Work out the finished part from the listing and answer in its coordinate system (mm). Face numbers are marked on the shaded views. A direction names the side the tool comes from. Round coordinates to 2 decimals unless told otherwise and drop trailing zeros. Order: outer loops, then holes, each group sorted by start corner. A loop starts at its lowest first (then second) coordinate and runs counter-clockwise, first axis right, second up. Notation, with made-up numbers: M 13,67.25 L 62,67.25 A30 ccw 62,97.25 Z; hole C 8,18.5 d8. An arc over 180 degrees is marked long. Answer as a JSON object with one key per item and string values. Group by question number.
from build123d import *

# Parameters (mm, degrees)
F0_R        = 1.7
F0_R_2      = 1.6
F1_DEPTH    = 10.4
F2_W        = 12.7
F2_H        = 2.7
F2_W_2      = 4
F2_H_2      = 1.35
F3_DEPTH    = 28
F4_W        = 12
F4_H        = 1.35
F5_DEPTH    = 6.2
F6_T1_DEPTH = 23.9048285752
F7_R        = 0.762


# Not quite as in the source:
# - a fillet or chamfer that OpenCascade refuses, or shapes differently, is made with other operations: its cross-section is extruded or revolved along the edge and cut away or added
# - a feature names something its author has since deleted; it is built from what else it names


with BuildPart() as f1:
    # F0 (on Top) → F1 (new body)
    with BuildSketch(Plane.XY):
        with BuildLine():
            Line((3.3782, 0), (0, 0))
            Line((0, 0), (0, -15.8))
            Line((0, -15.8), (15, -15.8))
            Line((15, -15.8), (15, -19.8))
            Line((15, -19.8), (27, -19.8))
            Line((27, -19.8), (27, -19))
            Line((27, -19), (15.8, -19))
            Line((15.8, -19), (15.8, -15.8))
            Line((15.8, -15.8), (28, -15.8))
            Line((28, -15.8), (28, -11))
            Line((28, -11), (40, -11))
            Line((40, -11), (40, -10.2))
            Line((40, -10.2), (28, -10.2))
            Line((28, -10.2), (28, -5.6))
            Line((28, -5.6), (40, -5.6))
            Line((40, -5.6), (40, -4.8))
            Line((40, -4.8), (28, -4.8))
            Line((28, -4.8), (28, 0))
            Line((28, 0), (6.1722, 0))
            Line((6.1722, 0), (6.1722, 1.345))
            ThreePointArc((6.1722, 1.345), (4.7752, 2.742), (3.3782, 1.345))
            Line((3.3782, 1.345), (3.3782, 0))
        make_face()
        with Locations((3.1, -13)):
            Circle(F0_R, mode=Mode.SUBTRACT)
        with Locations((25.3, -2.7)):
            Circle(F0_R_2, mode=Mode.SUBTRACT)
    extrude(amount=F1_DEPTH)

    # F2 (on face) → F3 (cut, through all)
    with BuildSketch(Plane(origin=(0, 0, 0), x_dir=(0, -1, 0), z_dir=(-1, 0, 0))):
        with Locations((-6.35, 9.05)):
            Rectangle(F2_W, F2_H)
        with Locations((-6.35, 1.35)):
            Rectangle(F2_W, F2_H)
        with Locations((17.8, 9.725)):
            Rectangle(F2_W_2, F2_H_2)
        with Locations((17.8, 0.675)):
            Rectangle(F2_W_2, F2_H_2)
    extrude(amount=-F3_DEPTH, mode=Mode.SUBTRACT)

    # F4 (on face) → F5 (cut, through all)
    with BuildSketch(Plane(origin=(0, -4.8, 0), x_dir=(-1, 0, 0), z_dir=(0, 1, 0))):
        with Locations((-34, 9.725)):
            Rectangle(F4_W, F4_H)
        with Locations((-34, 0.675)):
            Rectangle(F4_W, F4_H)
    extrude(amount=-F5_DEPTH, mode=Mode.SUBTRACT)

    # F6: fillet of radius 2.7 on 2 edges, made by hand

    # F6_s2 → F6_t1 (cut)
    with BuildSketch(Plane.XY.offset(-6.7524142876)):
        with BuildLine():
            ThreePointArc((25.2990343146, -15.8004), (27.2091883092, -15.0091883092), (28.0004, -13.0990343146))
            Line((28.0004, -13.0990343146), (28.2705365685, -13.0990343146))
            ThreePointArc((28.2705365685, -13.0990343146), (28.2701365685, -14.4495171573), (28.2701365685, -15.8))
            Line((28.2701365685, -15.8), (28, -16.0701365685))
            ThreePointArc((28, -16.0701365685), (26.6495171573, -16.0701365685), (25.2990343146, -16.0705365685))
            Line((25.2990343146, -16.0705365685), (25.2990343146, -15.8004))
        make_face()
    extrude(amount=F6_T1_DEPTH, mode=Mode.SUBTRACT)

    # F7
    f7_edges = [f1.edges().sort_by_distance(p)[0] for p in [
        (28, 0, 5.2),
        (0, -15.8, 5.2),
    ]]
    fillet(f7_edges, radius=F7_R)


solid = f1.part
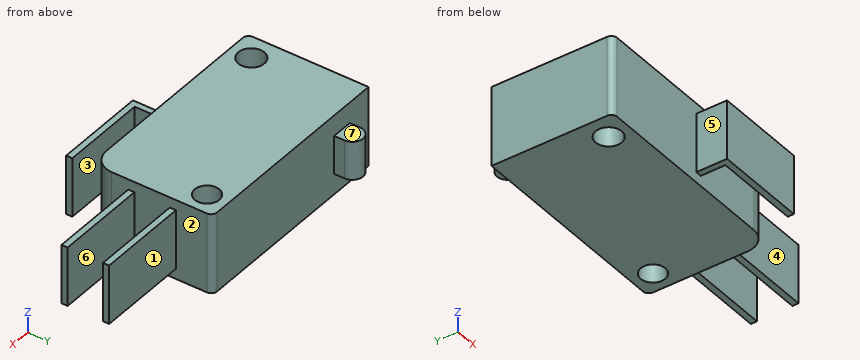
Item 1: Find section B-B (z = 7.25). Give the vertices of the cut face in (x, y) (3 decimals), and give its area (3 significant figures).
Item 2: The mould has two halves that part along Y. Classify the marked faces 1, 2, 3 and 4: +Y half, -Y half, draft (parallel to the pull), parting line (faces both ways), or undercut.
Item 3: Find section C-C (y = -2.7). Give the vertices of the cut face in (x, z), and give its area (3 significant figures).
Item 4: Each of these flat-tipped pins is pushed along its axis until it touches: pin 1 (2 mm diameter, centred on x = 9.5, z = 5.5, fed in from +Y); pin 2 (1.5 mm diameter, centred on x = 24, y = -16.5, fed in from -Z); pin 3 (0.6 mm diameter, centred on y = -19.5, z = 6, fed in from +X); pin 4 (1.4 mm diameter, centred on x = 4, y = 1, fed in from -Z). Where does it stop, or does it pass through?
Item 5: Consider L1, parallel to Y at x = 25.3, z = 2.75; L2, parallel to Y at x = 20, z = 6.75; L3, parallel to Y at x = 38, z = 4.5. Determine where each line is inside the solid, lowest interval first.
Item 6: Find section A-A (x = 31.5). Give the vertices of the cut face in (y, z), and give its area (3 significant figures).
Item 7: A tool of negligible diameter and unlimited length cuts with its end or side. For the marked faces 5, 6 and 7, from which of +Z, -Z, +X, -X, +Y, -Y can it reach the whole face along a straight path? Write none if from no direction.
Item 8: Find section D-D (y = -16.25). Give the vertices of the cut face in (x, z).
Responses:
{
 "1": {"outline": "M 0,-15.038 A0.762 ccw 0.762,-15.8 L 15,-15.8 L 15,-19.8 L 27,-19.8 L 27,-19 L 15.8,-19 L 15.8,-15.8 L 25.346,-15.8 A2.701 ccw 28,-13.146 L 28,-11 L 40,-11 L 40,-10.2 L 28,-10.2 L 28,-5.6 L 40,-5.6 L 40,-4.8 L 28,-4.8 L 28,-0.762 A0.762 ccw 27.238,0 L 6.172,0 L 6.172,1.345 A1.397 ccw 3.378,1.345 L 3.378,0 L 0,0 Z; hole C 3.1,-13 d3.4; hole C 25.3,-2.7 d3.2", "area": "462 mm^2"},
 "2": {"face 1": "+Y half", "face 2": "undercut", "face 3": "undercut", "face 4": "-Y half"},
 "3": {"outline": "M 0,0 L 23.7,0 L 23.7,10.4 L 0,10.4 Z; M 26.9,0 L 28,0 L 28,10.4 L 26.9,10.4 Z", "area": "258 mm^2"},
 "4": {"pin 1": "stops at y = 0", "pin 2": "stops at z = 0", "pin 3": "stops at x = 27", "pin 4": "stops at z = 2.7"},
 "5": {"L1": "y = -19.8 to -19, -15.8 to -4.3, -1.1 to 0", "L2": "y = -19.8 to -19, -15.8 to 0", "L3": "y = -11 to -10.2, -5.6 to -4.8"},
 "6": {"outline": "M -11,1.35 L -10.2,1.35 L -10.2,9.05 L -11,9.05 Z; M -5.6,1.35 L -4.8,1.35 L -4.8,9.05 L -5.6,9.05 Z", "area": "12.3 mm^2"},
 "7": {"face 5": "+Z, -Z, -X, -Y", "face 6": "+Z, -Z, +X", "face 7": "+Z, +X, -X, +Y"},
 "8": {"outline": "M 15,1.35 L 15.8,1.35 L 15.8,9.05 L 15,9.05 Z"}
}
